from build123d import *

# Parameters (mm, degrees)
PAD002_DEPTH             = 1
PAD003_DEPTH             = 0.25
BODY001_PLACEMENT_ANGLE  = 90
CLONE009_PLACEMENT_ANGLE = 180


with BuildPart() as part:
    # Sketch003 → Pad002 (new body)
    with BuildSketch(Plane.XY):
        with BuildLine():
            ThreePointArc((1.1456439239, -2.4999999999), (0, 2.75), (-1.1456439239, -2.4999999999))
            Line((-1.1456439239, -2.5), (1.1456439239, -2.5))
        make_face()
    extrude(amount=PAD002_DEPTH)

    # Sketch004 → Revolution001 (revolve)
    with BuildSketch(Plane.YZ):
        with BuildLine():
            add(Edge.make_bspline(
                [(-1.5494288107, 7.7), (-0.7747144053, 8.7), (0, 8.7)],
                knots=[-1.5494288107, -1.5494288107, -1.5494288107, 0, 0, 0], degree=2))
            Line((0, 8.7), (0, 1))
            Line((0, 1), (-2.5, 1))
            Line((-2.5, 1), (-2.3859606946, 5.3549853739))
            ThreePointArc((-2.3859606946, 5.3549853739), (-2.1547940918, 6.5942362206), (-1.5494288107, 7.7))
        make_face()
    revolve(axis=Axis((0, 0, 0), (0, 0, 1)))

    # Sketch005 → Pad003 (join, symmetric)
    with BuildSketch(Plane.YZ):
        Polygon((-1.52, 0), (-1.52, -2.9), (-1.82, -2.9), (-1.82, -4), (-1.52, -4), (-1.52, -7.175), (-1.02, -7.175), (-1.02, -4), (-0.72, -4), (-0.72, -2.9), (-1.02, -2.9), (-1.02, 0), align=None)
        Polygon((1.02, 0), (1.52, 0), (1.52, -2.9), (1.82, -2.9), (1.82, -4), (1.52, -4), (1.52, -8.175), (1.02, -8.175), (1.02, -4), (0.72, -4), (0.72, -2.9), (1.02, -2.9), align=None)
    extrude(amount=PAD003_DEPTH, both=True)


with BuildPart() as part_1:
    # Body001 placement: moved
    add(part.part.moved(Location((-3.81, 6.35, 4.445))).rotate(Axis((-3.81, 6.35, 4.445), (0, 0, -1)), BODY001_PLACEMENT_ANGLE))


with BuildPart() as part_2:
    # Clone009 placement: moved
    add(part_1.part.moved(Location((0, 12.7, 0))).rotate(Axis((0, 12.7, 0), (0, 0, 1)), CLONE009_PLACEMENT_ANGLE))


solid = part_2.part
The listing builds one solid part. Answer for the finished solid, in the listing's coordinates (mm). A direction names the side the tool comes from. Give positions to 0.01 mm unless a question says otherwise; leave off trailing zeros. Write each loop counter-clockwise with the first axis right and the second up, starting at its lowest first coordinate (ties: lowest second). Pieces come first, ordered by that corner, then holes. Notation, with made-up numbers: (3.5, -14.5) -> (22.5, -14.5) arc R25 cw to (22.5, 20.5) -> close; hole circle Ø2 at (84.25, -3). An arc over 180 degrees is marked (long way). One line per question, with ' | ' between items. Start each with the question number.
1. For faces 1 (the conical face through (3.49, 8.77, 7.65)), 2 (the flat face through (5, 6.1, 1)), 3 (the flat face through (2.5, 6.6, 0.4)), 4 (the cylindrical face through (1.06, 6.45, 4.94)), determine the directions among +Z, -Z, +X, -X, +Y, -Y from which every point of the face is accessible in a straight line to the end or side of a thin tool.
2. Find the intervals of material crossed by probe 1 along Z at (x, y) = (5.75, 4.7) (3 decimals); probe 2 along Y at (x, z) = (4.9, -1.25); probe 3 along X at (y, z) = (6.8, 11.25), in increasing order.
3. Section A-A (z = 2.5) is taken. Determine the outline of the cut face in (x, y).
4. Given pin 1 Ø1.6 at (x, y) = (4, 6.5) entering from -Z (3 decimals); pin 2 Ø1.6 at (x, y) = (3, 6.5) entering from +Z; pin 3 Ø3 at (y, z) = (8.5, 10) entering from +X; pin 4 Ø1.5 at (x, y) = (5, 7.5) entering from -Z (3 decimals), each flat-ended and moving along its own axis, determine where each tip first touches the part or whether it passes through.
Response values:
1) face 1: +Z | face 2: -Z, +X, -X, -Y | face 3: -Z, +X, -X, +Y | face 4: +Z, -Z
2) probe 1: 4.445 to 5.445 | probe 2: 6.1 to 6.6 | probe 3: 1.79 to 5.83
3) outline: (2.29, 6.1) -> (2.79, 6.1) -> (2.79, 6.6) -> (2.29, 6.6) -> close; (4.83, 6.1) -> (5.33, 6.1) -> (5.33, 6.6) -> (4.83, 6.6) -> close
4) pin 1: z = 0.445 | pin 2: z = 13.14 | pin 3: x = 6.1 | pin 4: z = 4.445
